```python
from build123d import *

# Parameters (mm, degrees)
EXTRUDE1_DEPTH = 3.81


with BuildPart() as part:
    # Sketch1 → Revolve1 (revolve)
    with BuildSketch(Plane.XY, mode=Mode.PRIVATE) as revolve1_sk:
        Polygon((28.702, 0), (28.702, 2.6035), (28.194, 3.1115), (-22.098, 3.1115), (-22.098, 4.826), (-28.194, 4.826), (-28.702, 4.318), (-28.702, 0), align=None)
    revolve(revolve1_sk.sketch.rotate(Axis((-40.759022879, 0, 0), (1, 0, 0)), 90), axis=Axis((-40.759022879, 0, 0), (1, 0, 0)))

    # Sketch2 → Extrude1 (cut)
    with BuildSketch(Plane.ZY.offset(28.702)):
        Polygon((0, 2.749630657), (-2.38125, 1.374815329), (-2.38125, -1.374815329), (0, -2.749630657), (2.38125, -1.374815329), (2.38125, 1.374815329), align=None)
    extrude(amount=-EXTRUDE1_DEPTH, mode=Mode.SUBTRACT)


solid = part.part
```
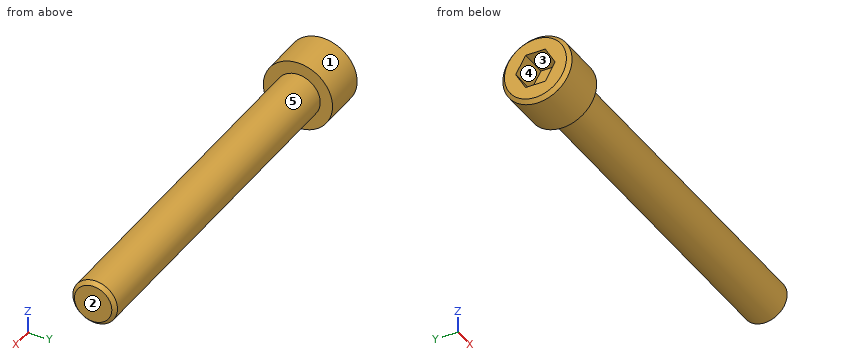
Input: part model. Units: mm. Frame: model coordinates. Face numbers are marked on the shaded views. A direction names the side the tool comes from. Coordinates: 2 decimals unless noted, no trailing zeros. Write each loop counter-clockwise with the first axis right and the second up, starting at its lowest first coordinate (ties: lowest second). Pieces come first, ordered by that corner, then holes.
1) Section B-B on x = -23. Output: boundary loops of the cut face in (y, z).
2) Set-up query: the marked faces 4 and 5. Return all of +Z, -Z, +X, -X, +Y, -Y with unobstructed straight access to the full face (end or side cutting, diameter ignored); none if empty.
3) Mould query, pull axis Z, two halves, no side actions, for the marked faces 1, 2 and 3. Classes: pulls with the +Z half, pulls with the -Z half, needs draft (parallel to the pull), parting line crosses it, or undercut.
4) Material intervals for line 1 along X through (y, z) = (-1.25, 0.5); line 2 along Z through (x, y) = (-0.5, -0.25); line 3 along Y through (x, z) = (-13.5, -2), sorted ascending.
5) Pin query (flat end, axial travel): pin 1 Ø1 at (x, y) = (-11, -1) entering from +Z; pin 2 Ø1.5 at (x, z) = (-2.5, 1) entering from +Y; pin 3 Ø4 at (x, y) = (16, 1.5) entering from -Z. Return the tip coordinate at first contact, or that it passes through.
6) Section C-C on x = 25. Output: boundary loops of the cut face in (y, z).
7) Section A-A on y = 0. Output: boundary loops of the cut face in (x, z), and give its area (3 significant figures).
Check result:
1. outline: circle Ø9.65 at (0, 0)
2. face 4: -X
2. face 5: +X
3. face 1: parting line crosses it
3. face 2: needs draft
3. face 3: undercut
4. line 1: x = -24.89 to 28.7
4. line 2: z = -3.1 to 3.1
4. line 3: y = -2.38 to 2.38
5. pin 1: stops at z = 3.07
5. pin 2: stops at y = 3.1
5. pin 3: stops at z = -3.11
6. outline: circle Ø6.22 at (0, 0)
7. outline: (-28.7, -4.32) - (-28.19, -4.83) - (-22.1, -4.83) - (-22.1, -3.11) - (28.19, -3.11) - (28.7, -2.6) - (28.7, 2.6) - (28.19, 3.11) - (-22.1, 3.11) - (-22.1, 4.83) - (-28.19, 4.83) - (-28.7, 4.32) - (-28.7, 2.38) - (-24.89, 2.38) - (-24.89, -2.38) - (-28.7, -2.38) - close
7. area: 361 mm2
